Input: part model. Units: mm. Frame: model coordinates. A direction names the side the tool comes from. Coordinates: 2 decimals unless noted, no trailing zeros. Loops run counter-clockwise (first coordinate to the right, second up) from the corner with the lowest first, then second, coordinate; pieces in that order, holes last. Notation, with made-up numbers: (50.25, 69) - (55.25, 69) arc R21 ccw to (55.25, 89) - close; hole circle Ø4 at (10, 17). An arc over 180 degrees is marked (long way). Use a Markdown table: item, result. Add a question column.
1. Access query for faces 3 (the face through (-112.705, -4.528, -2.535)), 4 (the face through (7.496, 0.232, -2.465)), 5 (the face through (-112.62, 4.5, -2.54)). Directions: +Z, -Z, +X, -X, +Y, -Y. A direction counts if a zero-diameter tool reaches every point of the face in a straight line with its end or side. Return the directions, or none.
2. Section query C-C on y = 0. Return the cut outline in (x, z).
3. Draft query along X for faces 1 (the face through (-61, 4, -2)), 2 (the face through (-59, 0, 0)). Return one class per face: released by +X, released by -X, zero draft, split by the parting line, or undercut.
4. Section query D-D on x = -65.5. Return the cut outline in (y, z).
5. Contact query for flat-ended pins moving along their axis: P1, Ø3, axis at y = 6, z = -4, coming from the +X side; P2, Ø3, axis at x = -104, z = -2, coming from the +Y side; P3, Ø1, axis at x = -114, z = -4, coming from the -Y side. Output: stop coordinate, or through.
6. Ray query, L1, parallel to X at y = 0.25, z = -4.3; L2, parallel to Y at x = 0, z = -1.05; L3, parallel to X at y = 0.75, z = -0.4. Return the intervals inside material, ascending. Write a range as [from, to].
7. Section query B-B on x = 0. Return the cut outline in (y, z).
8. Section query A-A on z = -3.1. Return the cut outline in (x, y).
```python
from build123d import *

# Parameters (mm, degrees)
SKETCH1_R          = 3.5
BASE_FLANGE1_DEPTH = 5
FILLET1_R          = 10


# Sheet-metal steps are written as plain solids
with BuildPart() as part:
    # Sketch1 → Base-Flange1 (new body)
    with BuildSketch(Plane.XY):
        with BuildLine():
            Line((-113.65571123, 4), (-6.34428877, 4))
            ThreePointArc((-6.34428877, 4), (7.5, 0), (-6.34428877, -4))
            Line((-6.34428877, -4), (-113.65571123, -4))
            ThreePointArc((-113.65571123, -4), (-127.5, 0), (-113.65571123, 4))
        make_face()
        with Locations((-120, 0)):
            Circle(SKETCH1_R, mode=Mode.SUBTRACT)
        Circle(SKETCH1_R, mode=Mode.SUBTRACT)
    extrude(amount=-BASE_FLANGE1_DEPTH)

    # Fillet1
    fillet1_edges = [part.edges().sort_by_distance(p)[0] for p in [
        (-113.65571123, 4, -2.5),
        (-6.34428877, 4, -2.5),
        (-6.34428877, -4, -2.5),
        (-113.65571123, -4, -2.5),
    ]]
    fillet(fillet1_edges, radius=FILLET1_R)


solid = part.part
```
Resolved:
| question | item | result |
|---|---|---|
| 1 | face 3 | +Z, -Z, -Y |
| 1 | face 4 | +Z, -Z |
| 1 | face 5 | +Z, -Z, +Y |
| 2 | outline | (-127.5, -5) - (-123.5, -5) - (-123.5, 0) - (-127.5, 0) - close; (-116.5, -5) - (-3.5, -5) - (-3.5, 0) - (-116.5, 0) - close; (3.5, -5) - (7.5, -5) - (7.5, 0) - (3.5, 0) - close |
| 3 | face 1 | undercut |
| 3 | face 2 | zero draft |
| 4 | outline | (-4, -5) - (4, -5) - (4, 0) - (-4, 0) - close |
| 5 | P1 | x = 6 |
| 5 | P2 | y = 4 |
| 5 | P3 | y = -5.34 |
| 6 | L1 | [-127.5, -123.49], [-116.51, -3.49], [3.49, 7.5] |
| 6 | L2 | [-7.5, -3.5], [3.5, 7.5] |
| 6 | L3 | [-127.46, -123.42], [-116.58, -3.42], [3.42, 7.46] |
| 7 | outline | (-7.5, -5) - (-3.5, -5) - (-3.5, 0) - (-7.5, 0) - close; (3.5, -5) - (7.5, -5) - (7.5, 0) - (3.5, 0) - close |
| 8 | outline | (-115.5, -6) arc R10 cw to (-109.5, -4) - (-10.5, -4) arc R10 cw to (-4.5, -6) arc R7.5 ccw (long way) to (-4.5, 6) arc R10 cw to (-10.5, 4) - (-109.5, 4) arc R10 cw to (-115.5, 6) arc R7.5 ccw (long way) to start; hole circle Ø7 at (-120, 0); hole circle Ø7 at (0, 0) |
